For this review, use the dimensioned drawing (mm, ordinates from the lowest corner) and the shaded views. A direction names the side the tool comes from. Round coordinates to 2 decimals unless told otherwise and drop trailing zeros. Write each loop counter-clockwise with the first axis right and the second up, starting at its lowest first coordinate (ties: lowest second). Pieces come first, ordered by that corner, then holes. Notation, with made-up numbers: (-5.5, 28) -> (49.5, 28) arc R20 ccw to (49.5, 34) -> close; hole circle Ø6 at (37.5, -0.5). An arc over 180 degrees is marked (long way). Answer in a Markdown table with one row per item. Add a question column.
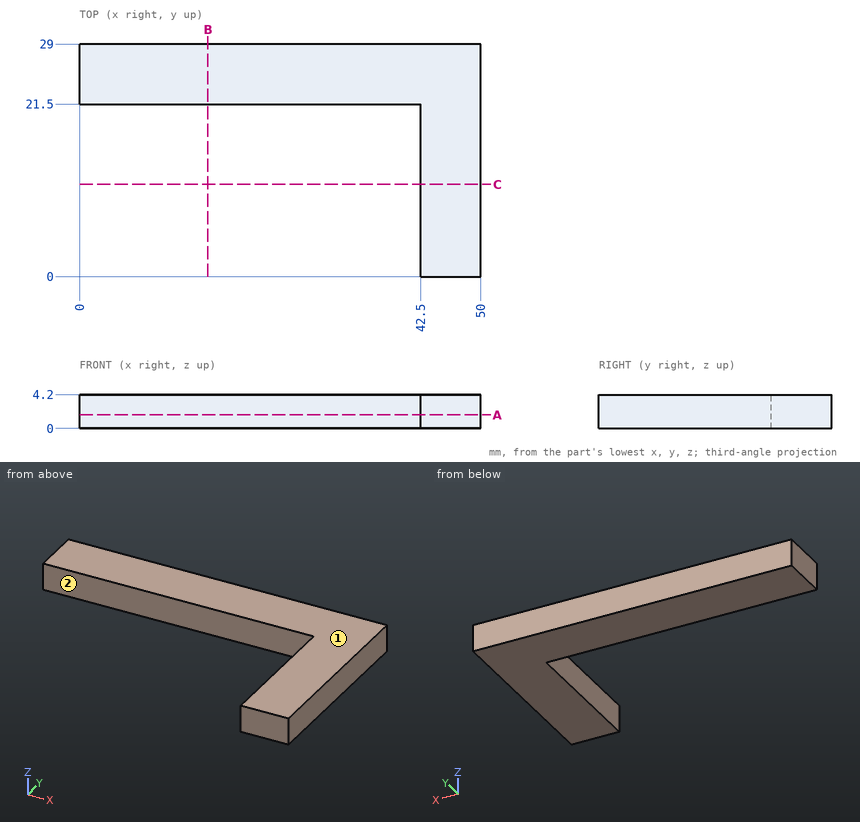
1. We need section C-C (y = 11.5). Write out the cut boundary in (x, z).
2. For L1, parallel to Y at x = 37.5, z = 1.65; L2, parallel to X at y = 20, z = 3.4, list the stretches that pass through material, from the lowest coordinate up. Write a range as [from, to].
3. We need section B-B (x = 16). Write out the cut boundary in (y, z), plus the area to 3 significant figures.
4. Clearance check with flat-ended pins moving along their axes: pin 1 Ø1.3 at (y, z) = (5.5, 2) entering from -X; pin 2 Ø3 at (x, y) = (19, 19.5) entering from -Z (1 decimal). State where each tip first meets the part, or that it passes through.
5. Tool access review of the marked faces 1 and 2: name each direction out of +Z, -Z, +X, -X, +Y, -Y from which nothing blocks a thin tool from reaching the whole face with its end or side.
6. We need section A-A (z = 1.7). Write out the cut boundary in (x, y).
Response:
| question | item | result |
|---|---|---|
| 1 | outline | (42.5, 0) -> (50, 0) -> (50, 4.2) -> (42.5, 4.2) -> close |
| 2 | L1 | [21.5, 29] |
| 2 | L2 | [42.5, 50] |
| 3 | outline | (21.5, 0) -> (29, 0) -> (29, 4.2) -> (21.5, 4.2) -> close |
| 3 | area | 31.5 mm2 |
| 4 | pin 1 | x = 42.5 |
| 4 | pin 2 | through |
| 5 | face 1 | +Z, +X, -X, +Y, -Y |
| 5 | face 2 | +Z, -Z, -X, -Y |
| 6 | outline | (0, 21.5) -> (42.5, 21.5) -> (42.5, 0) -> (50, 0) -> (50, 29) -> (0, 29) -> close |
